from build123d import *

# Parameters (mm, degrees)
CHAMFER1_SIZE     = 0.2
CIRPATTERN1_COUNT = 4


with BuildPart() as part:
    # Sketch1 → Revolve1 (revolve)
    with BuildSketch(Plane.XY, mode=Mode.PRIVATE) as revolve1_sk:
        Polygon((0, 5.1), (0, 11), (3.5, 11), (3.5, 5.1), (13.5, 5.1), (13.5, 3.5), (-1.5, 3.5), (-1.5, 5.1), align=None)
    revolve(revolve1_sk.sketch.rotate(Axis((0, 0, 0), (1, 0, 0)), 180), axis=Axis((0, 0, 0), (1, 0, 0)))

    # Chamfer1
    chamfer1_edges = [part.edges().sort_by_distance(p)[0] for p in [
        (-1.5, 3.5, 0),
        (13.5, 3.5, 0),
        (13.5, 5.1, 0),
        (3.5, 11, 0),
        (0, 11, 0),
        (-1.5, 5.1, 0),
    ]]
    chamfer(chamfer1_edges, length=CHAMFER1_SIZE)

    # Sketch5 → M3 Clearance Hole1 (revolve, cut)
    with BuildSketch(Plane(origin=(3.5, 8, 0), x_dir=(0, 0, -1), z_dir=(0, 1, 0))):
        Polygon((0, 0), (0, 4.051506083), (1.75, 3), (1.75, 0), align=None)
    m3_clearance_hole1 = revolve(axis=Axis((9.85, 8, 0), (-1, 0, 0)), mode=Mode.SUBTRACT)

    # CirPattern1: M3 Clearance Hole1 ×4 about axis
    cirpattern1_axis = Axis((0, 0, 0), (1, 0, 0))
    for i in range(1, CIRPATTERN1_COUNT):
        add(m3_clearance_hole1.rotate(cirpattern1_axis, i * 360 / CIRPATTERN1_COUNT), mode=Mode.SUBTRACT)


solid = part.part
Part model, mm, in its own coordinate system. A direction names the side the tool comes from. Round coordinates to 2 decimals unless told otherwise and drop trailing zeros. Write each loop counter-clockwise with the first axis right and the second up, starting at its lowest first coordinate (ties: lowest second). Pieces come first, ordered by that corner, then holes. Notation, with made-up numbers: M -35,27 L -9,27 A11 ccw -9,33 Z; hole C -9,41.5 d9. An arc over 180 degrees is marked long. Return JSON: item names as keys, results as strings. Group by question number.
(1) Drill centre lines: probe 1 along Z at (x, y) = (5.75, 0); probe 2 along X at (y, z) = (5.25, 7.75); probe 3 along Z at (x, y) = (11.5, -2). Where is each one in solid material? Low to high.
(2) Saw through at A-A on x = 11.25. Write the cut outline in (y, z), then the cut area to 3 significant figures.
(3) Which spindle directions (+Z, -Z, +X, -X, +Y, -Y) get a long thin tool onto all of the face, cutting with end or side? Do faces 5 (the face through (0, 5, 2)), 6 (the face through (-1.5, 1, -4)), 7 (the face through (8.469, -4.864, -1.532)). Say none if no direction does.
(4) Saw through at B-B on y = 0. Count the separate pieces of the cut face and the enclosed holes in it, then the cut area to 3 significant figures.
(5) Two-plate mould, pull along Y, no slides. Class faces 1 (the face through (2.021, 8.67, -1.617)), 2 (the face through (2.021, -8.67, 1.617)), 3 (the face through (13.5, -1, -4)), 4 (the face through (1.77, 2.38, 10.74)): +Y half, -Y half, draft (parallel to the pull), parting line (faces both ways), or undercut.
(6) Pin check, flat tips, straight feed: pin 1 Ø5.5 at (y, z) = (0, 8) entering from +X; pin 2 Ø8 at (x, z) = (10.5, 5.5) entering from -Y; pin 3 Ø3 at (y, z) = (8, 0) entering from -X. Stop position of each tip, or through.
Returned:
{
 "1": {"probe 1": "-5.1 to -3.5, 3.5 to 5.1", "probe 2": "0 to 3.5", "probe 3": "-4.69 to -2.87, 2.87 to 4.69"},
 "2": {"outline": "C 0,0 d10.2; hole C 0,0 d7", "area": "43.2 mm²"},
 "3": {"face 5": "-X", "face 6": "+Z, -Z, -X, +Y, -Y", "face 7": "+X"},
 "4": {"separate pieces": "4", "enclosed holes": "0", "area": "65.4 mm²"},
 "5": {"face 1": "undercut", "face 2": "undercut", "face 3": "draft", "face 4": "parting line"},
 "6": {"pin 1": "x = 3.5", "pin 2": "y = -4.87", "pin 3": "x = 0"}
}
